Input: part model. Units: mm. Frame: model coordinates. A direction names the side the tool comes from. Coordinates: 2 decimals unless noted, no trailing zeros. Write each loop counter-clockwise with the first axis right and the second up, starting at its lowest first coordinate (ties: lowest second). Pieces come first, ordered by that corner, then holes. Notation, with made-up numbers: M 31,9 L 58,9 A21 cw 58,14 Z; hole C -30.75,83 d10. An arc over 180 degrees is marked long. Write each question's results on one line, items separated by ' | '. Start each with the question number.
1. Set-up query: faces 1 (the flat face through (-1.2, -11.2, 4.6)), 2 (the cylindrical face through (6, 0.1, -0.5)), 3 (the flat face through (0, -5, 0)). Return all of +Z, -Z, +X, -X, +Y, -Y with unobstructed straight access to the full face (end or side cutting, diameter ignored); none if empty.
2. First-contact query: pin 1 (1.8 mm diameter, centred on x = 8, y = 0, fed in from +Z); pin 2 (4 mm diameter, centred on x = -2.5, y = 7.5, fed in from +Z). Flat tips, straight axial feed; report the tip coordinate or a pass-through.
3. Section query A-A, the plane x = -12.5. Output: boundary loops of the cut face in (y, z).
4. Section query D-D, the plane z = 1.2. Output: boundary loops of the cut face in (x, y), and give its area (3 significant figures).
5. Pull-direction query (X, two-part tool) for faces 4 (the cylindrical face through (-14, -12.43, 1.84)), 5 (the flat face through (15, 0, 2)), 6 (the flat face through (0, -15, 2)); classes: +X half, -X half, draft (parallel to the pull), parting line (faces both ways), or undercut.
6. Ray query, probe 1 along Y at (x, z) = (12.5, 1.15); probe 2 along X at (y, z) = (4.25, 1.8). Return the intervals inside material, ascending.
7. Section query C-C, the plane x = 1. Output: boundary loops of the cut face in (y, z).
```python
from build123d import *

# Parameters (mm, degrees)
CROQUIS1_W              = 30
CROQUIS1_H              = 30
CROQUIS1_R              = 1
SALIENTE_EXTRUIR2_DEPTH = 1
CROQUIS2_W              = 30
CROQUIS2_H              = 30
CROQUIS2_W_2            = 22
CROQUIS2_H_2            = 22
SALIENTE_EXTRUIR3_DEPTH = 10
CROQUIS4_R              = 1.5
CORTAR_EXTRUIR2_DEPTH   = 44
CROQUIS5_W              = 5.4
CROQUIS5_H              = 30
CORTAR_EXTRUIR3_DEPTH   = 46


with BuildPart() as part:
    # Croquis1 → Saliente-Extruir2 (new body)
    with BuildSketch(Plane.XY):
        Rectangle(CROQUIS1_W, CROQUIS1_H)
        with Locations((-8, 0)):
            Circle(CROQUIS1_R, mode=Mode.SUBTRACT)
        with Locations((8, 0)):
            Circle(CROQUIS1_R, mode=Mode.SUBTRACT)
        with BuildLine():
            Line((-1.75, 4.25), (1.75, 4.25))
            ThreePointArc((1.75, 4.25), (6, 0), (1.75, -4.25))
            Line((1.75, -4.25), (-1.75, -4.25))
            ThreePointArc((-1.75, -4.25), (-6, 0), (-1.75, 4.25))
        make_face(mode=Mode.SUBTRACT)
    extrude(amount=-SALIENTE_EXTRUIR2_DEPTH)

    # Croquis2 → Saliente-Extruir3 (add)
    with BuildSketch(Plane.XY):
        Rectangle(CROQUIS2_W, CROQUIS2_H)
        Rectangle(CROQUIS2_W_2, CROQUIS2_H_2, mode=Mode.SUBTRACT)
    extrude(amount=SALIENTE_EXTRUIR3_DEPTH)

    # Croquis4 → Cortar-Extruir2 (cut)
    with BuildSketch(Plane.XY.offset(10)):
        with Locations((-12.5, 12.5)):
            Circle(CROQUIS4_R)
        with Locations((12.5, 12.5)):
            Circle(CROQUIS4_R)
        with Locations((12.5, -12.5)):
            Circle(CROQUIS4_R)
        with Locations((-12.5, -12.5)):
            Circle(CROQUIS4_R)
    extrude(amount=-CORTAR_EXTRUIR2_DEPTH, mode=Mode.SUBTRACT)

    # Croquis5 → Cortar-Extruir3 (cut)
    with BuildSketch(Plane.ZY.offset(15)):
        with Locations((7.3, 0)):
            Rectangle(CROQUIS5_W, CROQUIS5_H)
    extrude(amount=-CORTAR_EXTRUIR3_DEPTH, mode=Mode.SUBTRACT)


solid = part.part
```
Answer:
1) face 1: +Z, +X, -X, +Y, -Y | face 2: +Z, -Z | face 3: +Z
2) pin 1: through | pin 2: z = 0
3) outline: M -15,-1 L -14,-1 L -14,4.6 L -15,4.6 Z; M -11,-1 L 11,-1 L 11,4.6 L -11,4.6 Z; M 14,-1 L 15,-1 L 15,4.6 L 14,4.6 Z
4) outline: M -15,-15 L 15,-15 L 15,15 L -15,15 Z; hole C -12.5,-12.5 d3; hole C -12.5,12.5 d3; hole M -11,-11 L 11,-11 L 11,11 L -11,11 Z; hole C 12.5,-12.5 d3; hole C 12.5,12.5 d3 | area: 388 mm^2
5) face 4: undercut | face 5: +X half | face 6: draft
6) probe 1: -15 to -14, -11 to 11, 14 to 15 | probe 2: -15 to -11, 11 to 15
7) outline: M -15,-1 L -4.25,-1 L -4.25,0 L -11,0 L -11,4.6 L -15,4.6 Z; M 4.25,-1 L 15,-1 L 15,4.6 L 11,4.6 L 11,0 L 4.25,0 Z
